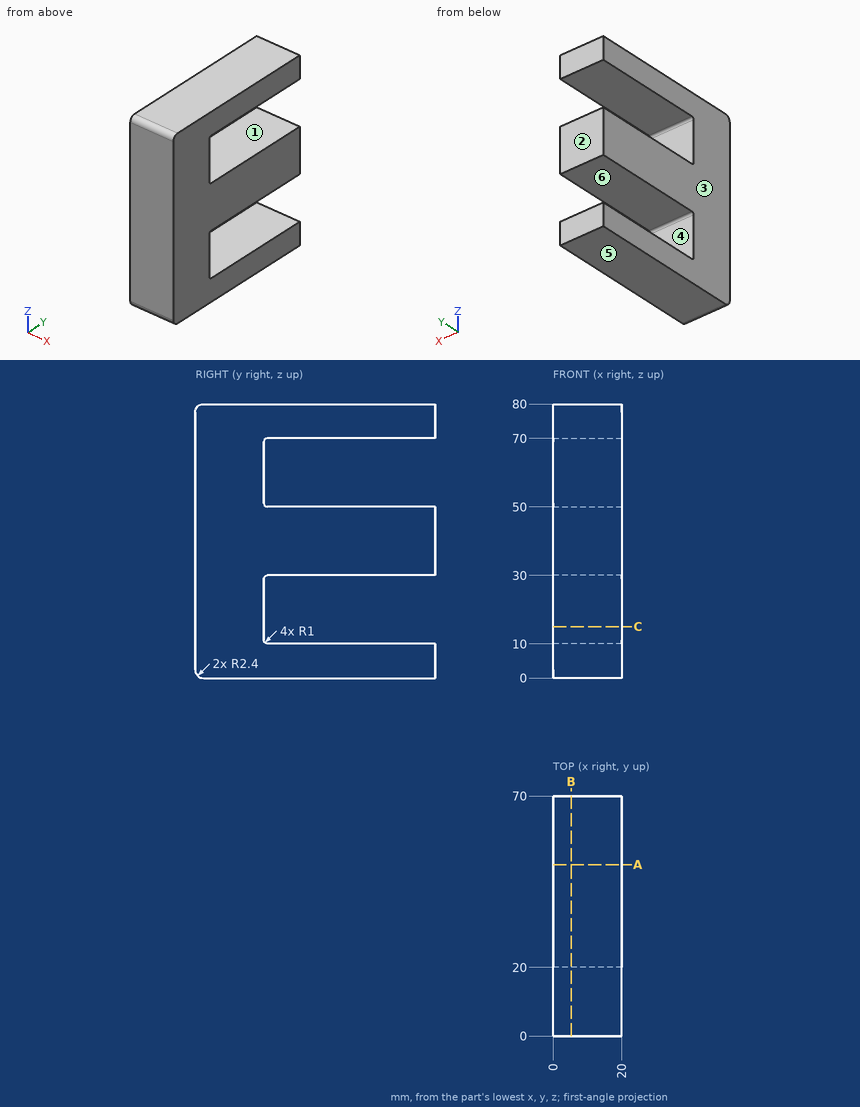
Verification items for this drawing (mm, ordinates from the low corner). A direction names the side the tool comes from. Round coordinates to 2 decimals unless told otherwise and drop trailing zeros. Loops run counter-clockwise (first coordinate to the right, second up) from the corner with the lowest first, then second, coordinate; pieces in that order, holes last. Notation, with made-up numbers: (71.25, -26.5) -> (103.25, -26.5) arc R34 ccw to (103.25, 6.5) -> close; hole circle Ø9 at (59, -36). An arc over 180 degrees is marked (long way). Write item = value, one per line. Start each with the question number.
1) Sectioned sample at B-B, the plane x = 5.25. Record the cut outline in (y, z), plus the area to 3 significant figures.
2) Sectioned sample at C-C, the plane z = 15. Record the cut outline in (x, y).
3) Set-up check for the marked faces 1 and 2: record each of +Z, -Z, +X, -X, +Y, -Y from which the full face is reachable in a straight line by a thin tool's end or side.
4) Thickness scan on probe 1 along Z at (x, y) = (18.25, 60.5); probe 2 along Y at (x, z) = (6.5, 65). Record the ranges inside material, lowest first.
5) Sectioned sample at A-A, the plane y = 50. Record the cut outline in (x, z), plus the area to 3 significant figures.
6) Release check for a two-part mould opening along Z. For the marked faces 3, 4, 5 and 6 record: released by +Z, released by -Z, zero draft, split by the parting line, or undercut.
Results are:
q1.outline = (0, 2.4) arc R2.4 ccw to (2.4, 0) -> (70, 0) -> (70, 10) -> (21, 10) arc R1 cw to (20, 11) -> (20, 29) arc R1 cw to (21, 30) -> (70, 30) -> (70, 50) -> (21, 50) arc R1 cw to (20, 51) -> (20, 69) arc R1 cw to (21, 70) -> (70, 70) -> (70, 80) -> (2.4, 80) arc R2.4 ccw to (0, 77.6) -> close
q1.area = 3,600 mm^2
q2.outline = (0, 0) -> (20, 0) -> (20, 20) -> (0, 20) -> close
q3.face_1 = +X, -X, +Y
q3.face_2 = +Z, -Z, +X, -X, +Y
q4.probe_1 = 0 to 10, 30 to 50, 70 to 80
q4.probe_2 = 0 to 20
q5.outline = (0, 0) -> (20, 0) -> (20, 10) -> (0, 10) -> close; (0, 30) -> (20, 30) -> (20, 50) -> (0, 50) -> close; (0, 70) -> (20, 70) -> (20, 80) -> (0, 80) -> close
q5.area = 800 mm^2
q6.face_3 = zero draft
q6.face_4 = undercut
q6.face_5 = released by -Z
q6.face_6 = undercut
